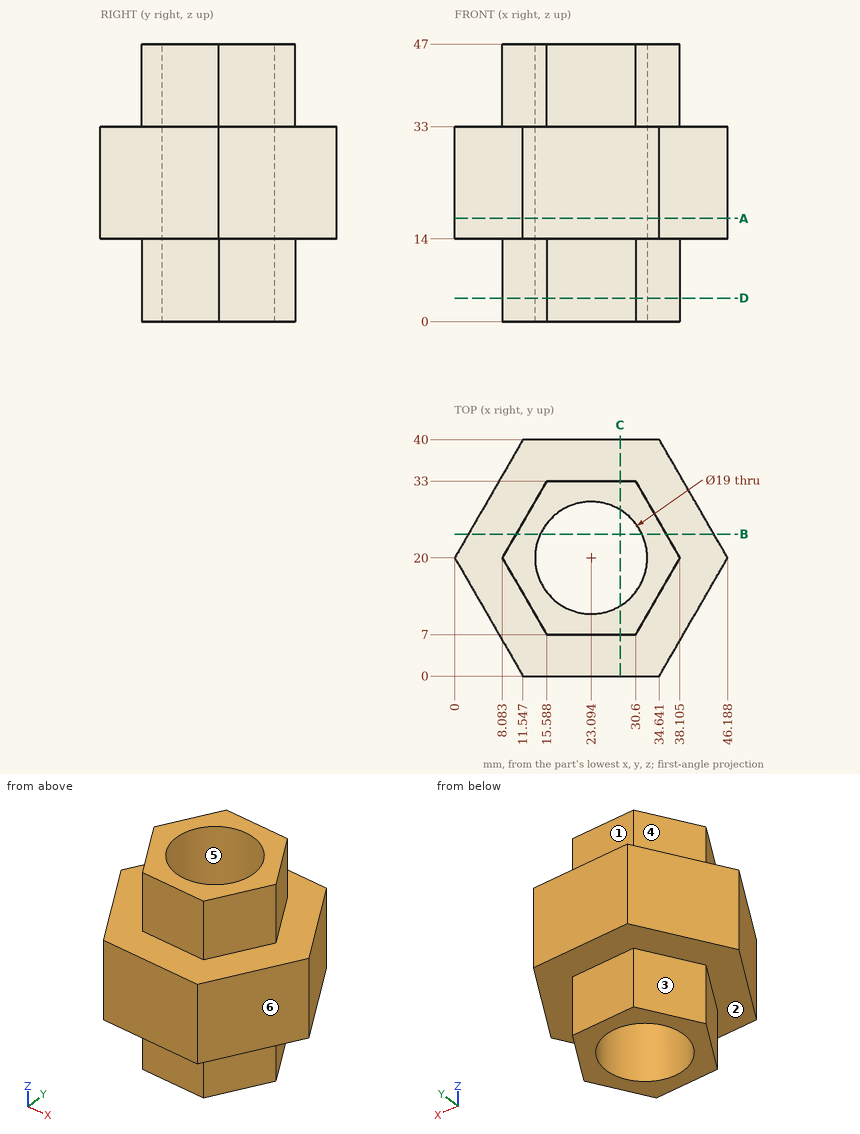
Can you work these out from the drawing? Everything is in mm from the part's minimum corner. A direction names the side the tool comes from. Give positions to 0.01 mm unless a question says otherwise; leave off trailing zeros. Order: outer loops, then holes, each group sorted by start corner. A loop starts at its lowest first (then second) coordinate and runs counter-clockwise, first axis right, second up. Notation, with made-up numbers: M 48.5,31.5 L 100.5,31.5 A37 ccw 100.5,69.5 Z; hole C -15,1 d10. An arc over 180 degrees is marked long. Use a Markdown table: item, result. Add a question column.
1. Suppose I cut it at A-A (z = 17.5). List the corners of the cut face in (x, y) for me, and give its area (3 significant figures).
2. On a 3-axis mill with a long thin cutter (end or side, diameter ignored), from which of +Z, -Z, +X, -X, +Y, -Y can I reach the whole of each face in a straight line? I mean the marked faces 1, 2 and 3. Say none if no direction works.
3. If we mould it in two halves opening along X, with no side actions, what happens to the marked faces 4, 5 and 6? For each: +X half, -X half, draft (parallel to the pull), parting line (faces both ways), or undercut.
4. Suppose I cut it at D-D (z = 4). List the corners of the cut face in (x, y) for me (1 decimal), and give its area (3 significant figures).
5. Suppose I cut it at B-B (y = 24). List the corners of the cut face in (x, z) for me (1 decimal), and give its area (3 significant figures).
6. For pin 1 Ø1.5 at (y, z) = (19, 21.5) entering from +X; pin 2 Ø3 at (y, z) = (18, 8.5) entering from -X; pin 3 Ø11 at (x, z) = (23.5, 6) entering from -Y; pin 4 Ø20 at (x, y) = (29, 19.5) entering from -Z, each with a flat end and sliding along its axis, tell me the tip position at first contact or that it passes through.
7. Suppose I cut it at C-C (x = 28). List the corners of the cut face in (y, z) for me (1 decimal).
8. I need wall thicknesses on probe 1 along Z at (x, y) = (7.5, 22); probe 2 along Y at (x, z) = (22.5, 39); probe 3 along Y at (x, z) = (16, 9.5). Which ranges of each line are inside material? Lowest first, please. Write a range as from..to.
Results list:
| question | item | result |
|---|---|---|
| 1 | outline | M 0,20 L 11.55,0 L 34.64,0 L 46.19,20 L 34.64,40 L 11.55,40 Z; hole C 23.09,20 d19 |
| 1 | area | 1,100 mm² |
| 2 | face 1 | +Z, +X, -X, +Y |
| 2 | face 2 | -Z |
| 2 | face 3 | -Z, -X, +Y |
| 3 | face 4 | -X half |
| 3 | face 5 | undercut |
| 3 | face 6 | +X half |
| 4 | outline | M 8.1,20 L 15.6,7 L 30.6,7 L 38.1,20 L 30.6,33 L 15.6,33 Z; hole C 23.1,20 d19 |
| 4 | area | 302 mm² |
| 5 | outline | M 2.3,14 L 10.4,14 L 10.4,0 L 14.5,0 L 14.5,47 L 10.4,47 L 10.4,33 L 2.3,33 Z; M 31.7,0 L 35.8,0 L 35.8,14 L 43.9,14 L 43.9,33 L 35.8,33 L 35.8,47 L 31.7,47 Z |
| 5 | area | 691 mm² |
| 6 | pin 1 | stops at x = 46.04 |
| 6 | pin 2 | stops at x = 8.37 |
| 6 | pin 3 | stops at y = 7 |
| 6 | pin 4 | stops at z = 0 |
| 7 | outline | M 0,14 L 7,14 L 7,0 L 11.9,0 L 11.9,47 L 7,47 L 7,33 L 0,33 Z; M 28.1,0 L 33,0 L 33,14 L 40,14 L 40,33 L 33,33 L 33,47 L 28.1,47 Z |
| 8 | probe 1 | z = 14..33 |
| 8 | probe 2 | y = 7..10.52, 29.48..33 |
| 8 | probe 3 | y = 7..13.68, 26.32..33 |
